For this review, take the finished solid that the model builds, in its own axes (mm). Give positions to 0.01 mm unless a question says otherwise; leave off trailing zeros. Order: outer loops, then holes, each group sorted by start corner. A loop starts at its lowest first (then second) coordinate and runs counter-clockwise, first axis right, second up. Notation, with made-up numbers: M -16.75,-6.5 L 14.25,-6.5 A19 ccw 14.25,-2.5 Z; hole C 0.25,41 d1. An arc over 180 degrees is marked long. Answer as CSV lines item,"result". Start each with the question number.
1. We need section A-A, the plane z = -45. Give the boundary of the cut face in (x, y).
2. We need section B-B, the plane y = 51. Give the boundary of the cut face in (x, z).
3. We need section C-C, the plane x = 485. Give the boundary of the cut face in (y, z), and give its area (3 significant figures).
4. For line 1 along Y through (x, z) = (723, -24); line 2 along Z through (x, y) = (1218.5, 93.5); line 3 along Z through (x, y) = (419, 140.5), list the stretches that pass through material, from the lowest coordinate up.
from build123d import *

# Parameters (mm, degrees)
SKETCH1_W               = 130
SKETCH1_H               = 130
EXTRUDE1_DEPTH          = 2000
CUT_EXTRUDE2_DEPTH      = 2012.218536112
CUT_EXTRUDE2_DEPTH_BACK = 2012.218536112


with BuildPart() as part:
    # Sketch1 → Extrude1 (new body)
    with BuildSketch(Plane(origin=(0, 0, 0), x_dir=(0, 0, -1), z_dir=(1, 0, 0))):
        with BuildLine():
            Line((10, 0), (140, 0))
            ThreePointArc((140, 0), (147.071067812, 2.928932188), (150, 10))
            Line((150, 10), (150, 140))
            ThreePointArc((150, 140), (147.071067812, 147.071067812), (140, 150))
            Line((140, 150), (10, 150))
            ThreePointArc((10, 150), (2.928932188, 147.071067812), (0, 140))
            Line((0, 140), (0, 10))
            ThreePointArc((0, 10), (2.928932188, 2.928932188), (10, 0))
        make_face()
        with Locations((75, 75)):
            Rectangle(SKETCH1_W, SKETCH1_H, mode=Mode.SUBTRACT)
    extrude(amount=EXTRUDE1_DEPTH)

    # Sketch2 → Cut-Extrude2 (cut, two sides: drawn at the far end of the back side and taken through both)
    with BuildSketch(Plane.XY.offset(-CUT_EXTRUDE2_DEPTH_BACK)):
        Polygon((3375.343105648, -3778.724126769), (2000, 0), (1945.40446486, 150), (570.061359213, 3928.724126769), (8127.509612751, 6679.410338064), (10932.791359186, -1028.037915474), align=None)
    extrude(amount=CUT_EXTRUDE2_DEPTH + CUT_EXTRUDE2_DEPTH_BACK, mode=Mode.SUBTRACT)


solid = part.part
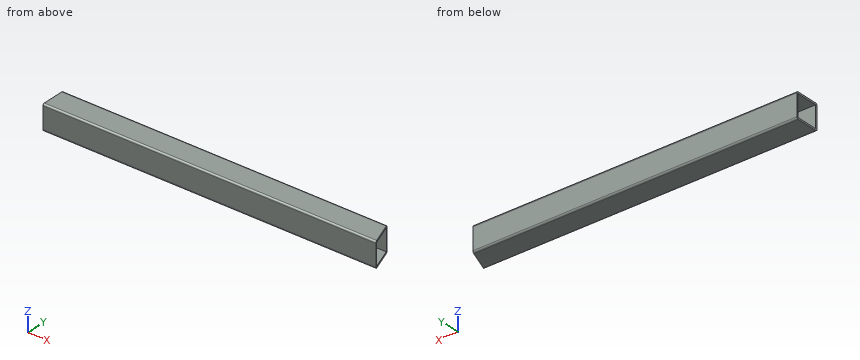
Result set:
1,outline,"M 0,0 L 2000,0 L 1996.36,10 L 0,10 Z; M 0,140 L 1949.04,140 L 1945.4,150 L 0,150 Z"
2,outline,"M 0,-150 L 1981.44,-150 L 1981.44,-140 L 0,-140 Z; M 0,-10 L 1981.44,-10 L 1981.44,0 L 0,0 Z"
3,outline,"M 0,-140 A10 ccw 10,-150 L 140,-150 A10 ccw 150,-140 L 150,-10 A10 ccw 140,0 L 10,0 A10 ccw 0,-10 Z; hole M 10,-140 L 140,-140 L 140,-10 L 10,-10 Z"
3,area,"5,510 mm2"
4,line 1,"0 to 10, 140 to 150"
4,line 2,"-150 to -140, -10 to 0"
4,line 3,"-149.99 to -0.01"
